Build history of the part. All positions in model axes, mm. Face numbers are marked on the shaded views. Round coordinates to 2 decimals unless told otherwise and drop trailing zeros. Loops run counter-clockwise (first coordinate to the right, second up) from the corner with the lowest first, then second, coordinate; pieces in that order, holes last. Notation, with made-up numbers: (18.5, -20) - (65.5, -20) arc R22 cw to (65.5, 11) - close; hole circle Ø4 at (51, 64.5). An arc over 180 degrees is marked (long way). Use a Markdown table: item, result.
from build123d import *

# Parameters (mm, degrees)
SKETCH_W                = 90
SKETCH_H                = 35
PAD_DEPTH               = 3
SKETCH001_R             = 10.5
HOLE_DEPTH              = 25
HOLE_TEARDROPS_DEPTH    = 25
SKETCH002_R             = 4
PAD001_DEPTH            = 5.6
POCKET_DEPTH            = 5.6
SKETCH004_R             = 1.45
HOLE001_DEPTH           = 25
HOLE001_TEARDROPS_DEPTH = 25
FILLET_R                = 2
CHAMFER_SIZE            = 0.4
FILLET001_R             = 1
CHAMFER001_SIZE         = 0.4


with BuildPart() as part:
    # Sketch → Pad (new body)
    with BuildSketch(Plane.XY):
        Rectangle(SKETCH_W, SKETCH_H)
    extrude(amount=PAD_DEPTH)

    # Sketch001 (on Face6 of Pad) → Hole (cut)
    with BuildSketch(Plane.XY.offset(3)):
        with Locations((-12, 0)):
            Circle(SKETCH001_R)
    extrude(amount=-HOLE_DEPTH, mode=Mode.SUBTRACT)

    # Sketch001_Teardrops (on Sketch) → Hole_Teardrops (cut)
    with BuildSketch(Plane.XY.offset(3)):
        with BuildLine():
            ThreePointArc((-17.25, 9.093267), (-12, -10.5), (-6.75, 9.093267))
            Line((-6.75, 9.093267), (-12, 12.124356))
            Line((-17.25, 9.093267), (-12, 12.124356))
        make_face()
    extrude(amount=-HOLE_TEARDROPS_DEPTH, mode=Mode.SUBTRACT)

    # Sketch002 (on Face5 of Hole_Teardrops) → Pad001 (join)
    with BuildSketch(Plane.XY.offset(3)):
        with Locations((35, 0)):
            Circle(SKETCH002_R)
        with Locations((12, 0)):
            Circle(SKETCH002_R)
        with Locations((-35, 0)):
            Circle(SKETCH002_R)
    extrude(amount=PAD001_DEPTH)

    # Sketch003 (on Face13 of Pad001) → Pocket (cut)
    with BuildSketch(Plane.XY.offset(8.6)):
        Polygon((-35, 3), (-38.464102, 5), (-31.535898, 5), align=None)
        Polygon((12, 3), (8.535898, 5), (15.464102, 5), align=None)
        Polygon((38.464102, 5), (35, 3), (31.535898, 5), align=None)
    extrude(amount=-POCKET_DEPTH, mode=Mode.SUBTRACT)

    # Sketch004 (on Face17 of Pocket) → Hole001 (cut)
    with BuildSketch(Plane.XY.offset(8.6)):
        with Locations((-35, 0)):
            Circle(SKETCH004_R)
        with Locations((12, 0)):
            Circle(SKETCH004_R)
        with Locations((35, 0)):
            Circle(SKETCH004_R)
    extrude(amount=-HOLE001_DEPTH, mode=Mode.SUBTRACT)

    # Sketch004_Teardrops (on Sketch) → Hole001_Teardrops (cut)
    with BuildSketch(Plane.XY.offset(8.6)):
        with BuildLine():
            ThreePointArc((-35.725, 1.255737), (-35, -1.45), (-34.275, 1.255737))
            Line((-34.275, 1.255737), (-35, 1.674316))
            Line((-35.725, 1.255737), (-35, 1.674316))
        make_face()
        with BuildLine():
            ThreePointArc((11.275, 1.255737), (12, -1.45), (12.725, 1.255737))
            Line((12.725, 1.255737), (12, 1.674316))
            Line((11.275, 1.255737), (12, 1.674316))
        make_face()
        with BuildLine():
            ThreePointArc((34.275, 1.255737), (35, -1.45), (35.725, 1.255737))
            Line((35.725, 1.255737), (35, 1.674316))
            Line((34.275, 1.255737), (35, 1.674316))
        make_face()
    extrude(amount=-HOLE001_TEARDROPS_DEPTH, mode=Mode.SUBTRACT)

    # Fillet
    fillet_edges = [part.edges().sort_by_distance(p)[0] for p in [
        (36.334875, 3.770691, 5.8),
        (33.665125, 3.770691, 5.8),
        (13.334875, 3.770691, 5.8),
        (10.665125, 3.770691, 5.8),
        (-33.665125, 3.770691, 5.8),
        (-36.334875, 3.770691, 5.8),
    ]]
    fillet(fillet_edges, radius=FILLET_R)

    # Chamfer
    chamfer_edges = [part.edges().sort_by_distance(p)[0] for p in [
        (33.392214, -3.662653, 8.6),
        (10.392214, -3.662653, 8.6),
        (-36.607786, -3.662653, 8.6),
        (-35.725, -1.255737, 8.6),
        (11.275, -1.255737, 8.6),
        (34.275, -1.255737, 8.6),
    ]]
    chamfer(chamfer_edges, length=CHAMFER_SIZE)

    # Fillet001
    fillet001_edges = [part.edges().sort_by_distance(p)[0] for p in [
        (45, 17.5, 1.5),
        (-45, 17.5, 1.5),
        (-45, -17.5, 1.5),
        (45, -17.5, 1.5),
    ]]
    fillet(fillet001_edges, radius=FILLET001_R)

    # Chamfer001
    chamfer001_edges = [part.edges().sort_by_distance(p)[0] for p in [
        (0, 17.5, 0),
        (0, 17.5, 3),
        (-35.725, -1.255737, 0),
        (-17.25, -9.093267, 0),
        (-17.25, -9.093267, 3),
        (11.275, -1.255737, 0),
        (34.275, -1.255737, 0),
    ]]
    chamfer(chamfer001_edges, length=CHAMFER001_SIZE)


solid = part.part
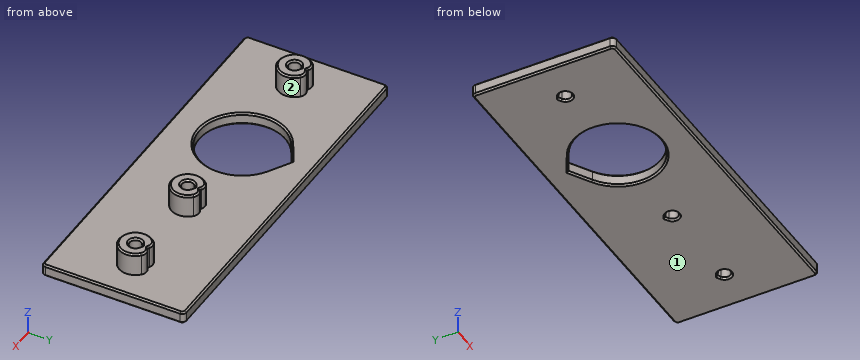
Q1. Drop flat-ended pins along their axis: pin 1 (3.5 mm diameter, centred on x = -35, y = 0, fed in from +Z); pin 2 (1.5 mm diameter, centred on y = -3.5, z = 5, fed in from +X); pin 3 (6 mm diameter, centred on x = -8.5, y = -9, fed in from +Z). Give the stop position or say it passes through.
Results found:
| item | result |
|---|---|
| pin 1 | stops at z = 8.5 |
| pin 2 | stops at x = 37.9 |
| pin 3 | stops at z = 3 |
Q2. Probe line 1 (X direction, y = 1.5, z = 1.75); line 2 (X direction, y = 0.5, z = 7.5); line 3 (Y direction, x = -12, z = 2.1). List the from-to ranges inside material, lowest first.
Results found:
| item | result |
|---|---|
| line 1 | x = -45 to -35.3, -34.7 to -22.39, -1.61 to 11.7, 12.3 to 34.7, 35.3 to 45 |
| line 2 | x = -38.97 to -36.36, -33.64 to -31.03, 8.03 to 10.64, 13.36 to 15.97, 31.03 to 33.64, 36.36 to 38.97 |
| line 3 | y = -17.5 to -10.5, 12.12 to 17.5 |
Q3. Pull direction X, two halves, no side cores. Call the marked faces 1 and 2: pulls with the +X half, pulls with the -X half, needs draft (parallel to the pull), parting line crosses it, or undercut.
Results found:
| item | result |
|---|---|
| face 1 | needs draft |
| face 2 | undercut |
Q4. Cut at C-C, the plane x = 0. List the corners of the cut face in (y, z).
Results found:
| item | result |
|---|---|
| outline | (-17.5, 0.4) - (-17.1, 0) - (17.1, 0) - (17.5, 0.4) - (17.5, 2.6) - (17.1, 3) - (-17.1, 3) - (-17.5, 2.6) - close |
Q5. Cut at B-B, the plane y = -13. List the corners of the cut face in (x, z).
Results found:
| item | result |
|---|---|
| outline | (-45, 0.4) - (-44.6, 0) - (44.6, 0) - (45, 0.4) - (45, 2.6) - (44.6, 3) - (-44.6, 3) - (-45, 2.6) - close |
Q6. Cut at A-A, the plane z = 4.5. List the corners of the cut face in (x, y) (3 decimals).
Results found:
| item | result |
|---|---|
| outline | (-37.708, 2.944) arc R4 ccw (long way) to (-32.292, 2.944) arc R2 ccw to (-34.646, 3.204) - (-35, 3) - (-35.354, 3.204) arc R2 ccw to start; (9.292, 2.944) arc R4 ccw (long way) to (14.708, 2.944) arc R2 ccw to (12.354, 3.204) - (12, 3) - (11.646, 3.204) arc R2 ccw to start; (32.292, 2.944) arc R4 ccw (long way) to (37.708, 2.944) arc R2 ccw to (35.354, 3.204) - (35, 3) - (34.646, 3.204) arc R2 ccw to start; hole (-35.725, 1.256) arc R1.45 ccw (long way) to (-34.275, 1.256) - (-35, 1.674) - close; hole (11.275, 1.256) arc R1.45 ccw (long way) to (12.725, 1.256) - (12, 1.674) - close; hole (34.275, 1.256) arc R1.45 ccw (long way) to (35.725, 1.256) - (35, 1.674) - close |
